Source: CAD feature listing. Evaluate the final solid. Frame: model axes, mm. Face numbers are marked on the shaded views. Round coordinates to 2 decimals unless told otherwise and drop trailing zeros. Loops run counter-clockwise (first coordinate to the right, second up) from the corner with the lowest first, then second, coordinate; pieces in that order, holes last. Notation, with made-up numbers: M -11,77.25 L 26,77.25 A17 ccw 26,90.25 Z; hole C 62.5,18 d8. An arc over 180 degrees is marked long. Answer as a JSON object with one key per item and string values.
Autodesk Inventor part; units mm, degrees
ref_plane "YZ Plane" through (0, 0, 0) normal (1, 0, 0) x (0, 1, 0)
ref_plane "XZ Plane" through (0, 0, 0) normal (0, 1, 0) x (-1, 0, 0)
ref_plane "XY Plane" through (0, 0, 0) normal (0, 0, 1) x (1, 0, 0)
sketch "Sketch1" plane through (0, 0, 0) normal (0, 0, 1) x (1, 0, 0)
  line L0 (-64, 31) -> (-73, 31)
  line L1 (-76, 28) -> (-76, 25)
  line L2 (-85, 16) -> (-76, 25)
  line L3 (-76, 28) -> (-73, 31)
  line L4 (-64, 31) -> (-55, 31)
  line L5 (-52, 28) -> (-52, 25)
  line L6 (-43, 16) -> (-52, 25)
  line L7 (-52, 28) -> (-55, 31)
  line L8 (-43, 16) -> (0, 16)
  line L9 (-77, 0) -> (-77, 5)
  line L10 (-77, 5) -> (-51, 5)
  line L11 (-51, 5) -> (-51, 0)
  line L12 (-106, 16) -> (-106, 7)
  line L13 (-106, 7) -> (-96, 7)
  line L14 (-96, 7) -> (-96, 16)
  line L15 (-128, 16) -> (-106, 16)
  line L16 (-96, 16) -> (-85, 16)
  line L17 (-120, 0) -> (-120, 7)
  line L18 (-120, 7) -> (-128, 7)
  line L19 (-120, 0) -> (-77, 0)
  line L20 (-128, 16) -> (-128, 7)
  line L21 (-8, 0) -> (-8, 7)
  line L22 (-8, 7) -> (0, 7)
  line L23 (-51, 0) -> (-8, 0)
  line L24 (0, 7) -> (0, 16)
  point P0 (0, 0)
  dimension "d0" = 128
  dimension "d6" = 3
  dimension "d67" = 5
  dimension "d71" = 22
  dimension "d74" = 9
  dimension "d75" = 10
  dimension "d93" = 7
  dimension "d94" = 8
  dimension "d95" = 7
extrude "Extrusion1" add sketch "Sketch1" against normal blind 2
sketch "Sketch2" plane through (0, 0, 0) normal (0, 0, 1) x (1, 0, 0)
  line L0 (-121, 10) -> (-125, 10)
  line L1 (-125, 10) -> (-125, 14)
  line L2 (-125, 14) -> (-121, 14)
  line L3 (-121, 14) -> (-121, 10)
  line L4 (-90, 0) -> (-80, 0)
  line L5 (-80, 0) -> (-80, 14)
  line L6 (-80, 14) -> (-90, 14)
  line L7 (-90, 14) -> (-90, 0)
  line L8 (-99, 1) -> (-103, 1)
  line L9 (-103, 1) -> (-103, 5)
  line L10 (-103, 5) -> (-99, 5)
  line L11 (-99, 5) -> (-99, 1)
  line L12 (-7, 10) -> (-3, 10)
  line L13 (-3, 10) -> (-3, 14)
  line L14 (-3, 14) -> (-7, 14)
  line L15 (-7, 14) -> (-7, 10)
  line L16 (-29, 1) -> (-25, 1)
  line L17 (-25, 1) -> (-25, 5)
  line L18 (-25, 5) -> (-29, 5)
  line L19 (-29, 5) -> (-29, 1)
  line L20 (-112, 13) -> (-120, 13)
  line L21 (-120, 13) -> (-120, 0)
  line L22 (-112, 13) -> (-112, 0)
  circle A0 centre (-123, 12) radius 1.25
  circle A1 centre (-101, 3) radius 1.25
  circle A2 centre (-27, 3) radius 1.25
  circle A3 centre (-5, 12) radius 1.25
  line L23 (-120, 0) -> (-112, 0)
  line L24 (-119.5, 12.5) -> (-119.5, 1.5)
  line L25 (-119.5, 1.5) -> (-112.5, 1.5)
  line L26 (-112.5, 1.5) -> (-112.5, 12.5)
  line L27 (-112.5, 12.5) -> (-119.5, 12.5)
  line L28 (-88.5, 12.5) -> (-88.5, 1.5)
  line L29 (-88.5, 1.5) -> (-81.5, 1.5)
  line L30 (-81.5, 1.5) -> (-81.5, 12.5)
  line L31 (-81.5, 12.5) -> (-88.5, 12.5)
  line L32 (-69, 14) -> (-59, 14)
  line L33 (-59, 14) -> (-59, 28)
  line L34 (-59, 28) -> (-69, 28)
  line L35 (-69, 28) -> (-69, 14)
  line L36 (-67.5, 26.5) -> (-67.5, 15.5)
  line L37 (-67.5, 15.5) -> (-60.5, 15.5)
  line L38 (-60.5, 15.5) -> (-60.5, 26.5)
  line L39 (-60.5, 26.5) -> (-67.5, 26.5)
  line L40 (-38, 0) -> (-48, 0)
  line L41 (-48, 0) -> (-48, 14)
  line L42 (-48, 14) -> (-38, 14)
  line L43 (-38, 14) -> (-38, 0)
  line L44 (-16, 13) -> (-8, 13)
  line L45 (-8, 13) -> (-8, 0)
  line L46 (-16, 13) -> (-16, 0)
  line L47 (-8, 0) -> (-16, 0)
  line L48 (-8.5, 12.5) -> (-8.5, 1.5)
  line L49 (-8.5, 1.5) -> (-15.5, 1.5)
  line L50 (-15.5, 1.5) -> (-15.5, 12.5)
  line L51 (-15.5, 12.5) -> (-8.5, 12.5)
  line L52 (-39.5, 12.5) -> (-39.5, 1.5)
  line L53 (-39.5, 1.5) -> (-46.5, 1.5)
  line L54 (-46.5, 1.5) -> (-46.5, 12.5)
  line L55 (-46.5, 12.5) -> (-39.5, 12.5)
  dimension "d49" = 2.5
  dimension "d50" = 2.5
  dimension "d51" = 2.5
  dimension "d52" = 2.5
  dimension "d69" = 13
sketch "Sketch10" plane through (0, 0, 0) normal (0, 0, 1) x (1, 0, 0)
  line L0 (-121, 10) -> (-125, 10)
  line L1 (-125, 10) -> (-125, 14)
  line L2 (-125, 14) -> (-121, 14)
  line L3 (-121, 14) -> (-121, 10)
  line L4 (-25, 1) -> (-25, 5)
  line L5 (-7, 14) -> (-7, 10)
  line L6 (-7, 10) -> (-3, 10)
  line L7 (-3, 10) -> (-3, 14)
  line L8 (-3, 14) -> (-7, 14)
  line L9 (-29, 1) -> (-25, 1)
  line L10 (-25, 5) -> (-29, 5)
  line L11 (-29, 5) -> (-29, 1)
  circle A0 centre (-123, 12) radius 1.25
  circle A1 centre (-27, 3) radius 1.25
  circle A2 centre (-5, 12) radius 1.25
  line L12 (-90, 0) -> (-80, 0)
  line L13 (-80, 0) -> (-80, 14)
  line L14 (-80, 14) -> (-90, 14)
  line L15 (-90, 14) -> (-90, 0)
  line L16 (-99, 1) -> (-103, 1)
  line L17 (-103, 1) -> (-103, 5)
  line L18 (-103, 5) -> (-99, 5)
  line L19 (-99, 5) -> (-99, 1)
  line L20 (-112, 13) -> (-120, 13)
  line L21 (-120, 13) -> (-120, 0)
  line L22 (-112, 13) -> (-112, 0)
  circle A3 centre (-101, 3) radius 1.25
  line L23 (-120, 0) -> (-112, 0)
  line L24 (-119.5, 12.5) -> (-119.5, 1.5)
  line L25 (-119.5, 1.5) -> (-112.5, 1.5)
  line L26 (-112.5, 1.5) -> (-112.5, 12.5)
  line L27 (-112.5, 12.5) -> (-119.5, 12.5)
  line L28 (-88.5, 12.5) -> (-88.5, 1.5)
  line L29 (-88.5, 1.5) -> (-81.5, 1.5)
  line L30 (-81.5, 1.5) -> (-81.5, 12.5)
  line L31 (-81.5, 12.5) -> (-88.5, 12.5)
  line L32 (-69, 14) -> (-59, 14)
  line L33 (-59, 14) -> (-59, 28)
  line L34 (-59, 28) -> (-69, 28)
  line L35 (-69, 28) -> (-69, 14)
  line L36 (-67.5, 26.5) -> (-67.5, 15.5)
  line L37 (-60.5, 26.5) -> (-67.5, 26.5)
  line L38 (-60.5, 15.5) -> (-60.5, 26.5)
  line L39 (-67.5, 15.5) -> (-60.5, 15.5)
  line L40 (-15.5, 1.5) -> (-15.5, 12.5)
  line L41 (-16, 13) -> (-16, 0)
  line L42 (-8.5, 1.5) -> (-15.5, 1.5)
  line L43 (-8, 0) -> (-16, 0)
  line L44 (-8.5, 12.5) -> (-8.5, 1.5)
  line L45 (-8, 13) -> (-8, 0)
  line L46 (-15.5, 12.5) -> (-8.5, 12.5)
  line L47 (-16, 13) -> (-8, 13)
  line L48 (-38, 0) -> (-48, 0)
  line L49 (-48, 0) -> (-48, 14)
  line L50 (-48, 14) -> (-38, 14)
  line L51 (-38, 14) -> (-38, 0)
  line L52 (-39.5, 12.5) -> (-39.5, 1.5)
  line L53 (-39.5, 1.5) -> (-46.5, 1.5)
  line L54 (-46.5, 1.5) -> (-46.5, 12.5)
  line L55 (-46.5, 12.5) -> (-39.5, 12.5)
  point P0 (-100.5385, 17.107)
  point P1 (-110.5385, 3.107)
  point P2 (-100.5385, 3.107)
  point P3 (-141.5385, 3.107)
  point P4 (-131.5385, 3.107)
  point P5 (-183.5385, 3.107)
  point P6 (-173.5385, 3.107)
  point P7 (-214.5385, 3.107)
  point P8 (-204.5385, 3.107)
  point P9 (-214.5385, 17.107)
  point P10 (0, 16)
  point P11 (0, 0)
  dimension "d62" = 2.5
  dimension "d64" = 2.5
  dimension "d65" = 2.5
extrude "Extrusion2" cut sketch "Sketch2" against normal blind 2 contours A0 | A1 | A2 | A3 | L27 L26 L25 L24 | L31 L30 L29 L28 | L39 L38 L37 L36 | L48 L49 L50 L51 | L52 L53 L54 L55
extrude "Extrusion7" add sketch "Sketch10" along normal blind 6
properties part number "Infravermelhos_revisto_2"
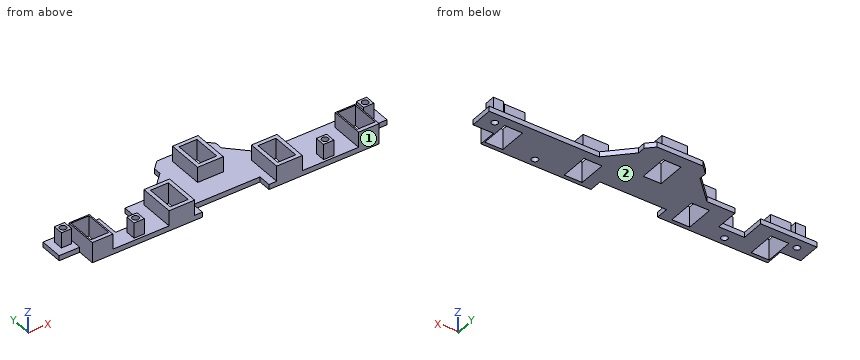
Item 1: Section D-D on y = 29.5. Return the cut outline in (x, z), then the cut area to 3 significant figures.
Answer sheet:
{"outline": "M -74.5,-2 L -53.5,-2 L -53.5,0 L -74.5,0 Z", "area": "42.0 mm²"}
Item 2: Section C-C on z = 3.5. Give the number of separate pieces and of enclosed holes in the cut face, then the cut area to 3 significant figures.
Answer sheet:
{"separate pieces": "9", "enclosed holes": "9", "area": "287 mm²"}
Item 3: Line query: probe 1 along Y at (x, z) = (-123, 3); probe 2 along X at (y, z) = (20, 2.5); probe 3 along X at (y, z) = (13.5, 5.5). Output: solid intervals per line, ascending. Write a range as from..to.
Answer sheet:
{"probe 1": "y = 10..10.75, 13.25..14", "probe 2": "x = -69..-67.5, -60.5..-59", "probe 3": "x = -125..-121, -90..-80, -48..-38, -7..-3"}
Item 4: Section B-B on x = -65. Return the cut outline in (y, z).
Answer sheet:
{"outline": "M 5,-2 L 15.5,-2 L 15.5,6 L 14,6 L 14,0 L 5,0 Z; M 26.5,-2 L 31,-2 L 31,0 L 28,0 L 28,6 L 26.5,6 Z"}
Item 5: Pull-direction query (Z, two-part tool) for the marked faces 1 and 2; classes: pulls with the +Z half, pulls with the -Z half, needs draft (parallel to the pull), parting line crosses it, or undercut.
Answer sheet:
{"face 1": "needs draft", "face 2": "pulls with the -Z half"}
Item 6: Section A-A on y = 21.5. Return the cut outline in (x, z), then the cut area to 3 significant figures.
Answer sheet:
{"outline": "M -79.5,-2 L -67.5,-2 L -67.5,6 L -69,6 L -69,0 L -79.5,0 Z; M -60.5,-2 L -48.5,-2 L -48.5,0 L -59,0 L -59,6 L -60.5,6 Z", "area": "66.0 mm²"}
Item 7: Contact query for flat-ended pins moving along their axis: pin 1 Ø1.8 at (x, z) = (-65.5, 2) entering from -Y; pin 2 Ø3 at (y, z) = (12.5, 3) entering from +X; pin 3 Ø1.8 at (x, z) = (-10.5, 4.5) entering from +Y; pin 4 Ø2.5 at (y, z) = (7, 0.5) entering from +X. Output: stop coordinate, or through.
Answer sheet:
{"pin 1": "stops at y = 14", "pin 2": "stops at x = -3", "pin 3": "stops at y = 13", "pin 4": "stops at x = 0"}
